Build history of the part. All positions in model axes, mm. A direction names the side the tool comes from. Coordinates: 2 decimals unless noted, no trailing zeros. Loops run counter-clockwise (first coordinate to the right, second up) from the corner with the lowest first, then second, coordinate; pieces in that order, holes last.
Item 1: Cut at D-D (z = 1.8). Count the separate pieces of the cut face and the enclosed holes in it, and give its area (3 significant figures).
Item 2: 3-axis set-ups, long thin cutter, end or side, ignore diameter. For faces 1 (the face through (44.475, -63.019, 2.535)), 2 (the face through (-71.95, -22.42, 2.46)): which of +Z, -Z, +X, -X, +Y, -Y reach the whole face in a straight line?
Item 3: Cut at B-B (x = -83). List the corners of the cut face in (y, z), and give its area (3 significant figures).
Item 4: Cut at C-C (y = -63.5). List the corners of the cut face in (x, z), and give its area (3 significant figures).
Item 5: Mould opens along Y. For faces 3 (the face through (-180.424, -1, 2)), 4 (the face through (-70.37, -33, 3)), 5 (the face through (-64, -73, 2)) say: released by +Y, released by -Y, zero draft, split by the parting line, or undercut.
Item 6: Cut at A-A (y = 0). List the corners of the cut face in (x, z), and give its area (3 significant figures).
Item 7: Drill centre lines: line 1 along X through (y, z) = (35.5, 3.9); line 2 along Y through (x, z) = (-115, 1.5); line 3 along X through (y, z) = (-11, 3.7). Where is each one in solid material? Low to high.
Item 8: Flat gauge pins, fed straight in: pin 1 (5 mm diameter, centred on x = -70.37, y = -8.66, fed in from +Z); pin 2 (3 mm diameter, centred on x = 15.63, y = -34.3, fed in from -Z). Where does each tip first touch, or does it go through?
from build123d import *

# Parameters (mm, degrees)
SKETCH_1_R          = 2.6
SKETCH_1_R_2        = 2.55
SKETCH_1_R_3        = 1.6
SKETCH_1_R_4        = 1.55
SKETCH_1_R_5        = 28
EXTRUDE_2_DEPTH     = 5
CUT_EXTRUDE_1_DEPTH = 10
SKETCH_4_R          = 1.6
SKETCH_4_R_2        = 1.55
CUT_EXTRUDE_2_DEPTH = 10
SKETCH_6_R          = 1.55
CUT_EXTRUDE_3_DEPTH = 10
FILLET_4_R          = 3
FILLET_5_R          = 3
FILLET_6_R          = 3
FILLET_7_R          = 3
FILLET_8_R          = 3
FILLET_9_R          = 3
FILLET_10_R         = 5
FILLET_11_R         = 5
FILLET_12_R         = 5


with BuildPart() as part:
    # 草图1 → 凸台-拉伸2 (new body)
    with BuildSketch(Plane.XY):
        Polygon((-63, 73), (47, 73), (55, 73), (55, -73), (47, -73), (-173, -73), (-180.424412423, -73), (-180.424412423, 73), (-172.424412423, 73), align=None)
        with Locations((-101.5, 63.5)):
            Circle(SKETCH_1_R, mode=Mode.SUBTRACT)
        with Locations((-63, 63.5)):
            Circle(SKETCH_1_R, mode=Mode.SUBTRACT)
        with Locations((-24.5, 63.5)):
            Circle(SKETCH_1_R, mode=Mode.SUBTRACT)
        with Locations((-24.5, -63.5)):
            Circle(SKETCH_1_R_2, mode=Mode.SUBTRACT)
        with Locations((-63, -63.5)):
            Circle(SKETCH_1_R, mode=Mode.SUBTRACT)
        with Locations((-101.5, -63.5)):
            Circle(SKETCH_1_R, mode=Mode.SUBTRACT)
        with Locations((-128.856103106, 36.5)):
            Circle(SKETCH_1_R_3, mode=Mode.SUBTRACT)
        with Locations((-152.317850859, 27.960622174)):
            Circle(SKETCH_1_R_3, mode=Mode.SUBTRACT)
        with Locations((-164.801586091, 6.338158485)):
            Circle(SKETCH_1_R_3, mode=Mode.SUBTRACT)
        with Locations((-160.466030344, -18.25)):
            Circle(SKETCH_1_R_3, mode=Mode.SUBTRACT)
        with Locations((-141.339838337, -34.298780659)):
            Circle(SKETCH_1_R_3, mode=Mode.SUBTRACT)
        with Locations((-116.372367874, -34.298780659)):
            Circle(SKETCH_1_R_3, mode=Mode.SUBTRACT)
        with Locations((-105.394355352, 27.960622174)):
            Circle(SKETCH_1_R_3, mode=Mode.SUBTRACT)
        with Locations((-92.910620121, 6.338158485)):
            Circle(SKETCH_1_R_3, mode=Mode.SUBTRACT)
        with Locations((-97.246175868, -18.25)):
            Circle(SKETCH_1_R_3, mode=Mode.SUBTRACT)
        with Locations((3.143896894, 36.5)):
            Circle(SKETCH_1_R_4, mode=Mode.SUBTRACT)
        with Locations((-20.317850859, 27.960622174)):
            Circle(SKETCH_1_R_3, mode=Mode.SUBTRACT)
        with Locations((-32.801586091, 6.338158485)):
            Circle(SKETCH_1_R_3, mode=Mode.SUBTRACT)
        with Locations((-28.466030344, -18.25)):
            Circle(SKETCH_1_R_3, mode=Mode.SUBTRACT)
        with Locations((-9.339838337, -34.298780659)):
            Circle(SKETCH_1_R_3, mode=Mode.SUBTRACT)
        with Locations((15.627632126, -34.298780659)):
            Circle(SKETCH_1_R_3, mode=Mode.SUBTRACT)
        with Locations((34.753824132, -18.25)):
            Circle(SKETCH_1_R_3, mode=Mode.SUBTRACT)
        with Locations((39.089379879, 6.338158485)):
            Circle(SKETCH_1_R_3, mode=Mode.SUBTRACT)
        with Locations((26.605644648, 27.960622174)):
            Circle(SKETCH_1_R_3, mode=Mode.SUBTRACT)
        with Locations((-128.856103106, 0)):
            Circle(SKETCH_1_R_5, mode=Mode.SUBTRACT)
        with Locations((3.143896894, 0)):
            Circle(SKETCH_1_R_5, mode=Mode.SUBTRACT)
    extrude(amount=EXTRUDE_2_DEPTH)

    # 草图3 → 切除-拉伸1 (cut)
    with BuildSketch(Plane.XY.offset(5)):
        with BuildLine():
            Line((-180.424412423, 73), (-180.424412423, 38))
            ThreePointArc((-180.424412423, 38), (-170.173149765, 62.748737342), (-145.424412423, 73))
            Line((-145.424412423, 73), (-180.424412423, 73))
        make_face()
        with BuildLine():
            Line((-180.424412423, -73), (-180.424412423, -38))
            ThreePointArc((-180.424412423, -38), (-170.173149765, -62.748737342), (-145.424412423, -73))
            Line((-145.424412423, -73), (-180.424412423, -73))
        make_face()
        with BuildLine():
            Line((55, 73), (20, 73))
            ThreePointArc((20, 73), (44.748737342, 62.748737342), (55, 38))
            Line((55, 38), (55, 73))
        make_face()
        with BuildLine():
            Line((55, -38), (55, -73))
            Line((55, -73), (20, -73))
            ThreePointArc((20, -73), (44.748737342, -62.748737342), (55, -38))
        make_face()
    extrude(amount=-CUT_EXTRUDE_1_DEPTH, mode=Mode.SUBTRACT)

    # 草图4 → 切除-拉伸2 (cut)
    with BuildSketch(Plane.XY.offset(5)):
        with Locations((-70.36973236, 21.338158485)):
            Circle(SKETCH_4_R)
        with Locations((-55.342473852, 21.338158485)):
            Circle(SKETCH_4_R)
        with Locations((-70.36973236, -8.661841515)):
            Circle(SKETCH_4_R)
        with Locations((-55.342473852, -8.661841515)):
            Circle(SKETCH_4_R_2)
    extrude(amount=-CUT_EXTRUDE_2_DEPTH, mode=Mode.SUBTRACT)

    # 草图6 → 切除-拉伸3 (cut)
    with BuildSketch(Plane.XY.offset(5)):
        with Locations((-62.856103106, 6.338158485)):
            Circle(SKETCH_6_R)
        Polygon((-82.36973236, 28.338158485), (-87.36973236, 28.338158485), (-62.856103106, 50.070242379), (-38.342473852, 28.338158485), (-43.342473852, 28.338158485), align=None)
        Polygon((-70.36973236, -19.661841515), (-70.36973236, -47.040526198), (-92.36973236, -33.351183857), align=None)
        Polygon((-55.342473852, -19.661841515), (-55.342473852, -47.040526198), (-33.342473852, -33.351183857), align=None)
    extrude(amount=-CUT_EXTRUDE_3_DEPTH, mode=Mode.SUBTRACT)

    # 圆角4
    fillet_4_edges = [part.edges().sort_by_distance(p)[0] for p in [
        (-70.36973236, -19.661841515, 2.5),
    ]]
    fillet(fillet_4_edges, radius=FILLET_4_R)

    # 圆角5
    fillet_5_edges = [part.edges().sort_by_distance(p)[0] for p in [
        (-92.36973236, -33.351183857, 2.5),
    ]]
    fillet(fillet_5_edges, radius=FILLET_5_R)

    # 圆角6
    fillet_6_edges = [part.edges().sort_by_distance(p)[0] for p in [
        (-70.36973236, -47.040526198, 2.5),
    ]]
    fillet(fillet_6_edges, radius=FILLET_6_R)

    # 圆角7
    fillet_7_edges = [part.edges().sort_by_distance(p)[0] for p in [
        (-55.342473852, -47.040526198, 2.5),
    ]]
    fillet(fillet_7_edges, radius=FILLET_7_R)

    # 圆角8
    fillet_8_edges = [part.edges().sort_by_distance(p)[0] for p in [
        (-55.342473852, -19.661841515, 2.5),
    ]]
    fillet(fillet_8_edges, radius=FILLET_8_R)

    # 圆角9
    fillet_9_edges = [part.edges().sort_by_distance(p)[0] for p in [
        (-33.342473852, -33.351183857, 2.5),
    ]]
    fillet(fillet_9_edges, radius=FILLET_9_R)

    # 圆角10
    fillet_10_edges = [part.edges().sort_by_distance(p)[0] for p in [
        (-62.856103106, 50.070242379, 2.5),
    ]]
    fillet(fillet_10_edges, radius=FILLET_10_R)

    # 圆角11
    fillet_11_edges = [part.edges().sort_by_distance(p)[0] for p in [
        (-87.36973236, 28.338158485, 2.5),
    ]]
    fillet(fillet_11_edges, radius=FILLET_11_R)

    # 圆角12
    fillet_12_edges = [part.edges().sort_by_distance(p)[0] for p in [
        (-38.342473852, 28.338158485, 2.5),
    ]]
    fillet(fillet_12_edges, radius=FILLET_12_R)


solid = part.part
Filled sheet:
1. separate pieces: 1
1. enclosed holes: 34
1. area: 27,100 mm2
2. face 1: +Z, -Z, +X, -Y
2. face 2: +Z, -Z
3. outline: (-73, 0) - (-39.18, 0) - (-39.18, 5) - (-73, 5) - close; (-27.52, 0) - (73, 0) - (73, 5) - (-27.52, 5) - close
3. area: 672 mm2
4. outline: (-169.4, 0) - (-104.1, 0) - (-104.1, 5) - (-169.4, 5) - close; (-98.9, 0) - (-65.6, 0) - (-65.6, 5) - (-98.9, 5) - close; (-60.4, 0) - (-27.05, 0) - (-27.05, 5) - (-60.4, 5) - close; (-21.95, 0) - (43.97, 0) - (43.97, 5) - (-21.95, 5) - close
4. area: 989 mm2
5. face 3: zero draft
5. face 4: undercut
5. face 5: released by -Y
6. outline: (-180.42, 0) - (-156.86, 0) - (-156.86, 5) - (-180.42, 5) - close; (-100.86, 0) - (-24.86, 0) - (-24.86, 5) - (-100.86, 5) - close; (31.14, 0) - (55, 0) - (55, 5) - (31.14, 5) - close
6. area: 617 mm2
7. line 1: x = -180.42 to -130.11, -127.61 to -78.7, -47.01 to 1.96, 4.33 to 55
7. line 2: y = -73 to -35.12, -33.48 to -24.33, 24.33 to 73
7. line 3: x = -180.42 to -154.6, -103.11 to -22.6, 28.89 to 55
8. pin 1: stops at z = 5
8. pin 2: passes through
